Can you work these out from the model? Positions are in its coordinate system, mm. Face numbers are marked on the shaded views. A direction names the side the tool comes from. Coordinates: 2 decimals unless noted, no trailing zeros. Order: outer loops, then holes, each group sorted by start corner. A loop starts at its lowest first (then second) coordinate and runs counter-clockwise, first axis right, second up. Notation, with made-up numbers: (44, 31.5) - (56, 31.5) arc R19 ccw to (56, 51.5) - close; hole circle Ø5 at (54.25, 64.25). An arc over 180 degrees is marked (long way). Return JSON: item names as keys, results as strings. Group by question number.
1) If we mould it in two halves opening along Z, with no side actions, what happens to the marked faces 1, 2 and 3? For each: pulls with the +Z half, pulls with the -Z half, needs draft (parallel to the pull), parting line crosses it, or undercut.
2) Imagine slicing it at A-A (z = 0.5). Write out the boundary of the cut face in (x, y), and give its area (3 significant figures).
3) For pin 1 Ø2 at (x, y) = (-4.25, 7.36) entering from +Z; pin 2 Ø5 at (x, z) = (-3.5, 14) entering from -Y; pin 3 Ø5 at (x, y) = (-1, 2) entering from +Z, each with a flat end and sliding along its axis, tell me the tip position at first contact or that it passes through.
4) Which directions (+Z, -Z, +X, -X, +Y, -Y) give clear straight access to the entire face, cutting with the end or side of a thin tool? Please do the marked faces 4, 5 and 6.
5) Imagine slicing it at C-C (z = 7.5). Write out the boundary of the cut face in (x, y).
6) Imagine slicing it at B-B (z = 33). Write out the boundary of the cut face in (x, y), and give its area (3 significant figures).
7) If I drill on line 1 along Y through (x, z) = (0, 1.8); line 2 along Y through (x, z) = (0, 25.25); line 3 along Z through (x, y) = (-10.75, 1.25), over which ranges is the centre line in solid material (lowest first)?
```python
from build123d import *

# Parameters (mm, degrees)
ESQUISSE1_R             = 15
EXTRUSION1_DEPTH        = 35.1
ESQUISSE2_R             = 9
EXTRUSION2_DEPTH        = 4
ESQUISSE3_R             = 5
EXTRUSION3_DEPTH        = 0.5
CHANFREIN1_SIZE         = 1
ENL_V_MAT_EXTRU_1_REACH = 6.5
ESQUISSE7_R             = 4
ESQUISSE8_R             = 15
ESQUISSE8_R_2           = 14.9
ENL_V_MAT_EXTRU_2_DEPTH = 20
ESQUISSE9_R             = 15
EXTRUSION4_DEPTH        = 5
TROU_TARAUD_M31_D       = 2.5
TROU_TARAUD_M31_DEPTH   = 4.5
TROU_TARAUD_M31_TIP     = 0.751075774
ESQUISSE10_R            = 5
ENL_V_MAT_EXTRU_3_DEPTH = 15
D_GAGEMENT_M21_D        = 2.4
D_GAGEMENT_M21_DEPTH    = 3
D_GAGEMENT_M21_TIP      = 0.721032743


with BuildPart() as part:
    # Esquisse1 → Extrusion1 (new body)
    with BuildSketch(Plane.XY):
        Circle(ESQUISSE1_R)
    extrude(amount=EXTRUSION1_DEPTH)

    # Esquisse2 → Extrusion2 (add)
    with BuildSketch(Plane(origin=(0, 0, 0), x_dir=(-1, 0, 0), z_dir=(0, 0, -1))):
        Circle(ESQUISSE2_R)
    extrude(amount=EXTRUSION2_DEPTH)

    # Esquisse3 → Extrusion3 (add)
    with BuildSketch(Plane(origin=(0, 0, -4), x_dir=(-1, 0, 0), z_dir=(0, 0, -1))):
        Circle(ESQUISSE3_R)
    extrude(amount=EXTRUSION3_DEPTH)

    # Chanfrein1
    chanfrein1_edges = [part.edges().sort_by_distance(p)[0] for p in [
        (-15, 0, 35.1),
    ]]
    chamfer(chanfrein1_edges, length=CHANFREIN1_SIZE)

    # Esquisse7 → Enlèv. mat.-Extru.1 (cut, up to next)
    with BuildSketch(Plane(origin=(0, 0, 0), x_dir=(-1, 0, 0), z_dir=(0, 0, -1)), mode=Mode.PRIVATE) as enl_v_mat_extru_1_sk1:
        Circle(ESQUISSE7_R)
    enl_v_mat_extru_1_tool1 = extrude(enl_v_mat_extru_1_sk1.sketch, amount=ENL_V_MAT_EXTRU_1_REACH, mode=Mode.PRIVATE) & part.part
    add(enl_v_mat_extru_1_tool1.solids().sort_by_distance((0, 0, 0))[0], mode=Mode.SUBTRACT)

    # Esquisse8 → Enlèv. mat.-Extru.2 (cut)
    with BuildSketch(Plane(origin=(0, 0, 0), x_dir=(-1, 0, 0), z_dir=(0, 0, -1))):
        Circle(ESQUISSE8_R)
        Circle(ESQUISSE8_R_2, mode=Mode.SUBTRACT)
    extrude(amount=-ENL_V_MAT_EXTRU_2_DEPTH, mode=Mode.SUBTRACT)

    # Esquisse9 → Extrusion4 (add)
    with BuildSketch(Plane(origin=(0, 0, 0), x_dir=(-1, 0, 0), z_dir=(0, 0, -1))):
        Circle(ESQUISSE9_R)
    extrude(amount=-EXTRUSION4_DEPTH)

    # Trou taraudé M31
    with Locations(Plane(origin=(0, 0, 0), x_dir=(-1, 0, 0), z_dir=(0, 0, -1))):
        with Locations((13, 0), (0, 13), (-13, 0), (0, -13)):
            Hole(TROU_TARAUD_M31_D / 2, depth=TROU_TARAUD_M31_DEPTH)
            with Locations((0, 0, -(TROU_TARAUD_M31_DEPTH + TROU_TARAUD_M31_TIP / 2))):  # 118° drill point
                Cone(0, TROU_TARAUD_M31_D / 2, TROU_TARAUD_M31_TIP, mode=Mode.SUBTRACT)

    # Esquisse10 → Enlèv. mat.-Extru.3 (cut)
    with BuildSketch(Plane.XY.offset(35.1)):
        Circle(ESQUISSE10_R)
    extrude(amount=-ENL_V_MAT_EXTRU_3_DEPTH, mode=Mode.SUBTRACT)

    # Dégagement M21
    with Locations(Plane.XY.offset(35.1)):
        with Locations((4.25, -7.361215932), (-4.25, -7.361215932), (-8.5, 0), (-4.25, 7.361215932), (4.25, 7.361215932), (8.5, 0)):
            Hole(D_GAGEMENT_M21_D / 2, depth=D_GAGEMENT_M21_DEPTH)
            with Locations((0, 0, -(D_GAGEMENT_M21_DEPTH + D_GAGEMENT_M21_TIP / 2))):  # 118° drill point
                Cone(0, D_GAGEMENT_M21_D / 2, D_GAGEMENT_M21_TIP, mode=Mode.SUBTRACT)


solid = part.part
```
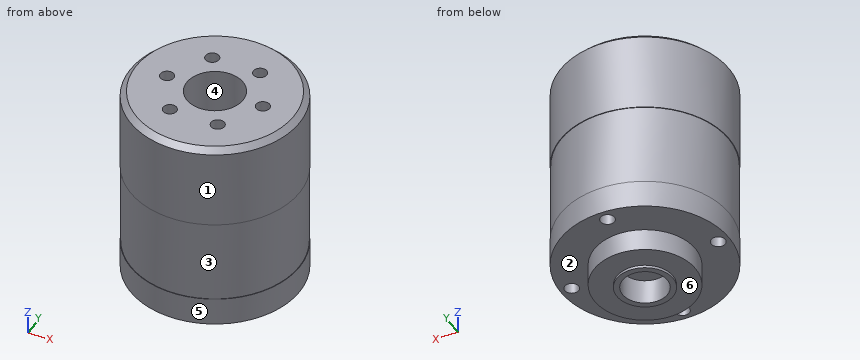
Calculated:
{
 "1": {"face 1": "needs draft", "face 2": "pulls with the -Z half", "face 3": "undercut"},
 "2": {"outline": "circle Ø30 at (0, 0); hole circle Ø2.5 at (-13, 0); hole circle Ø2.5 at (0, -13); hole circle Ø2.5 at (0, 13); hole circle Ø2.5 at (13, 0)", "area": "687 mm2"},
 "3": {"pin 1": "z = 31.98", "pin 2": "y = -14.87", "pin 3": "z = 20.1"},
 "4": {"face 4": "+Z", "face 5": "+Z, -Z", "face 6": "-Z"},
 "5": {"outline": "circle Ø29.8 at (0, 0)"},
 "6": {"outline": "circle Ø30 at (0, 0); hole circle Ø2.4 at (-8.5, 0); hole circle Ø2.4 at (-4.25, -7.36); hole circle Ø2.4 at (-4.25, 7.36); hole circle Ø10 at (0, 0); hole circle Ø2.4 at (4.25, -7.36); hole circle Ø2.4 at (4.25, 7.36); hole circle Ø2.4 at (8.5, 0)", "area": "601 mm2"},
 "7": {"line 1": "-15 to -14.25, -11.75 to 11.75, 14.25 to 15", "line 2": "-15 to -5, 5 to 15", "line 3": "0 to 35.1"}
}
